```python
from build123d import *

# Parameters (mm, degrees)
BOSS_EXTRUDE1_DEPTH = 40
SKETCH2_W           = 2.5
SKETCH2_H           = 2
BOSS_EXTRUDE2_DEPTH = 2
FILLET1_R           = 1


with BuildPart() as part:
    # Sketch1 → Boss-Extrude1 (new body)
    with BuildSketch(Plane(origin=(0, 0, 0), x_dir=(1, 0, 0), z_dir=(0, 1, 0))):
        Polygon((26.5, 2), (-26.5, 2), (-26.5, -4), (-22, -4), (-22, -2), (-24.5, -2), (-24.5, 0), (24.5, 0), (24.5, -2), (22, -2), (22, -4), (26.5, -4), align=None)
    extrude(amount=BOSS_EXTRUDE1_DEPTH)

    # Sketch2 → Boss-Extrude2 (add)
    with BuildSketch(Plane(origin=(0, 0, 0), x_dir=(1, 0, 0), z_dir=(0, 1, 0))):
        with Locations((-23.25, -1)):
            Rectangle(SKETCH2_W, SKETCH2_H)
        with Locations((23.25, -1)):
            Rectangle(SKETCH2_W, SKETCH2_H)
    extrude(amount=BOSS_EXTRUDE2_DEPTH)

    # Fillet1
    fillet1_edges = [part.edges().sort_by_distance(p)[0] for p in [
        (22, 20, 4),
        (26.5, 20, 4),
        (26.5, 20, -2),
        (-26.5, 20, -2),
        (-26.5, 20, 4),
        (-22, 20, 4),
    ]]
    fillet(fillet1_edges, radius=FILLET1_R)


solid = part.part
```
CAD build for the part. Positions are in the model's coordinates, mm. A direction names the side the tool comes from. Coordinates: 2 decimals unless noted, no trailing zeros. Order: outer loops, then holes, each group sorted by start corner. A loop starts at its lowest first (then second) coordinate and runs counter-clockwise, first axis right, second up. Notation, with made-up numbers: M 44,77.5 L 88,77.5 A19 cw 88,96.5 Z; hole C 64,59 d11. An arc over 180 degrees is marked long. Write each question's results on one line, items separated by ' | '. Start each with the question number.
Q1. Cut at C-C (x = -18). List the corners of the cut face in (y, z), then the cut area to 3 significant figures.
Q2. Which spindle directions (+Z, -Z, +X, -X, +Y, -Y) get a long thin tool onto all of the face, cutting with end or side? Do faces 4 (the flat face through (-0.4, 0, -0.4)), 5 (the flat face through (-23, 21, 2)), 6 (the flat face through (-22, 15.3, 2.2)). Say none if no direction does.
Q3. Pull direction X, two halves, no side cores. Call faces 1 (the flat face through (26.5, 20, 1)), 2 (the flat face through (24, 20, 4)), 3 (the flat face through (-23, 2, 1)): +X half, -X half, draft (parallel to the pull), parting line (faces both ways), or undercut.
Q4. Flat gauge pins, fed straight in: P1, Ø2, axis at x = 15.5, y = 6.5, coming from the +Z side; P2, Ø3, axis at x = -20.5, z = -0.5, coming from the -Y side; P3, Ø1.6, axis at x = 23, z = 1, coming from the +Y side. Where does each tip first touch, or does it go through?
Q5. Drill centre lines: probe 1 along X at (y, z) = (10, 0.1); probe 2 along Z at (x, y) = (8.5, 25.5); probe 3 along X at (y, z) = (37.5, 2.4). Where is each one in solid material? Low to high. Write a range as from..to.
Q6. Cut at A-A (z = 0.65). List the corners of the cut face in (x, y), then the cut area to 3 significant figures.
Q7. Cut at B-B (y = 26). List the corners of the cut face in (x, z), then the cut area to 3 significant figures.
Found:
1) outline: M 0,-2 L 40,-2 L 40,0 L 0,0 Z | area: 80.0 mm²
2) face 4: +Z, -Z, +X, -X, -Y | face 5: +Y | face 6: +Z, +Y, -Y
3) face 1: +X half | face 2: draft | face 3: undercut
4) P1: z = 0 | P2: y = 0 | P3: y = 2
5) probe 1: -26.5..-24.5, 24.5..26.5 | probe 2: -2..0 | probe 3: -26.5..-22, 22..26.5
6) outline: M -26.5,0 L -22,0 L -22,2 L -24.5,2 L -24.5,40 L -26.5,40 Z; M 22,0 L 26.5,0 L 26.5,40 L 24.5,40 L 24.5,2 L 22,2 Z | area: 170 mm²
7) outline: M -26.5,-1 A1 ccw -25.5,-2 L 25.5,-2 A1 ccw 26.5,-1 L 26.5,3 A1 ccw 25.5,4 L 23,4 A1 ccw 22,3 L 22,2 L 24.5,2 L 24.5,0 L -24.5,0 L -24.5,2 L -22,2 L -22,3 A1 ccw -23,4 L -25.5,4 A1 ccw -26.5,3 Z | area: 131 mm²
